from build123d import *

# Parameters (mm, degrees)
SKETCH_1_W          = 16
SKETCH_1_H          = 26
EXTRUDE_1_DEPTH     = 5
CUT_EXTRUDE_START   = 1
SKETCH_2_W          = 14
SKETCH_2_H          = 25
CUT_EXTRUDE_1_DEPTH = 10
EXTRUDE_START       = 5
SKETCH_3_W          = 16
SKETCH_3_H          = 26
EXTRUDE_3_DEPTH     = 1
CUT_EXTRUDE_START_2 = 6
SKETCH_4_W          = 14
SKETCH_4_H          = 17
CUT_EXTRUDE_2_DEPTH = 1
SKETCH_5_W          = 16
SKETCH_5_H          = 26
CUT_EXTRUDE_3_DEPTH = 1


with BuildPart() as part:
    # 스케치1 → 보스-돌출1 (new body)
    with BuildSketch(Plane(origin=(0, 0, 0), x_dir=(1, 0, 0), z_dir=(0, 1, 0))):
        Rectangle(SKETCH_1_W, SKETCH_1_H)
    extrude(amount=EXTRUDE_1_DEPTH)

    # 스케치2 → 컷-돌출1 (cut)
    with BuildSketch(Plane(origin=(0, 0, 0), x_dir=(1, 0, 0), z_dir=(0, 1, 0)).offset(CUT_EXTRUDE_START)):
        with Locations((0, 0.5)):
            Rectangle(SKETCH_2_W, SKETCH_2_H)
    extrude(amount=CUT_EXTRUDE_1_DEPTH, mode=Mode.SUBTRACT)


with BuildPart() as body_2:
    # 스케치3 → 보스-돌출3 (new body)
    with BuildSketch(Plane(origin=(0, 0, 0), x_dir=(1, 0, 0), z_dir=(0, 1, 0)).offset(EXTRUDE_START)):
        Rectangle(SKETCH_3_W, SKETCH_3_H)
    extrude(amount=EXTRUDE_3_DEPTH)

    # 스케치4 → 컷-돌출2 (cut)
    with BuildSketch(Plane(origin=(0, 0, 0), x_dir=(1, 0, 0), z_dir=(0, 1, 0)).offset(CUT_EXTRUDE_START_2)):
        with Locations((0, -1.5)):
            Rectangle(SKETCH_4_W, SKETCH_4_H)
    extrude(amount=-CUT_EXTRUDE_2_DEPTH, mode=Mode.SUBTRACT)

    # 스케치5 → 컷-돌출3 (cut)
    with BuildSketch(Plane(origin=(0, 6, 0), x_dir=(1, 0, 0), z_dir=(0, 1, 0))):
        Rectangle(SKETCH_5_W, SKETCH_5_H)
    extrude(amount=-CUT_EXTRUDE_3_DEPTH, mode=Mode.SUBTRACT)


solid = part.part
Verification items for the finished model (mm, model axes). A direction names the side the tool comes from. Give positions to 0.01 mm unless a question says otherwise; leave off trailing zeros. Write each loop counter-clockwise with the first axis right and the second up, starting at its lowest first coordinate (ties: lowest second). Pieces come first, ordered by that corner, then holes. Notation, with made-up numbers: (-25, -15.75) - (-18, -15.75) arc R32 cw to (-18, 11.25) - close; hole circle Ø11 at (20, 12). An arc over 180 degrees is marked (long way). Answer as CSV lines item,"result". Start each with the question number.
1. Sectioned sample at C-C (x = 2.25). Record the boundary of the cut face in (y, z), then the cut area to 3 significant figures.
2. Draft check along X on faces 3 (the face through (-7.15, 5, 2.83)), 4 (the face through (-7, 3, 0)), 5 (the face through (-8, 2, 0)). Enter one of: pulls with the +X half, pulls with the -X half, needs draft (parallel to the pull), parting line crosses it, or undercut.
3. Thickness scan on line 1 (X direction, y = 1.9, z = 5.25); line 2 (Z direction, x = 3, y = 1.9); line 3 (Y direction, x = -4.25, z = 4). Record the ranges inside material, lowest first.
4. Sectioned sample at A-A (y = 4.25). Record the boundary of the cut face in (x, z), then the cut area to 3 significant figures.
5. Sectioned sample at B-B (z = 8.75). Record the boundary of the cut face in (x, y).
6. Depth check by flat-ended pin: pin 1 (1.2 mm diameter, centred on x = -3.5, y = 3.5, fed in from -Z). Enter the tip coordinate at first touch or a pass-through.
7. Set-up check for faces 1 (the face through (7, 3, 0)), 2 (the face through (8, 2, 0)): record each of +Z, -Z, +X, -X, +Y, -Y from which the full face is reachable in a straight line by a thin tool's end or side.
Derived:
1,outline,"(0, -13) - (1, -13) - (1, 12) - (5, 12) - (5, 13) - (0, 13) - close"
1,area,"30.0 mm²"
2,face 3,"needs draft"
2,face 4,"undercut"
2,face 5,"pulls with the -X half"
3,line 1,"-8 to -7, 7 to 8"
3,line 2,"12 to 13"
3,line 3,"0 to 1"
4,outline,"(-8, -13) - (-7, -13) - (-7, 12) - (7, 12) - (7, -13) - (8, -13) - (8, 13) - (-8, 13) - close"
4,area,"66.0 mm²"
5,outline,"(-8, 0) - (8, 0) - (8, 5) - (7, 5) - (7, 1) - (-7, 1) - (-7, 5) - (-8, 5) - close"
6,pin 1,"z = 12"
7,face 1,"-Z, +Y"
7,face 2,"+Z, -Z, +X, +Y, -Y"
